```python
from build123d import *

# Parameters (mm, degrees)
SKETCH1_R           = 57.15
SKETCH1_R_2         = 48.26
BOSS_EXTRUDE1_DEPTH = 8.89
SKETCH1_4_R         = 57.15
SKETCH1_4_R_2       = 48.26
BOSS_EXTRUDE2_DEPTH = 177.8
FILLET1_R           = 5


with BuildPart() as part:
    # Sketch1 → Boss-Extrude1 (new body)
    with BuildSketch(Plane(origin=(0, 0, 0), x_dir=(1, 0, 0), z_dir=(0, 1, 0))):
        with Locations(Location((0, 0, 0), (0, 0, 90))):
            Circle(SKETCH1_R)
        Circle(SKETCH1_R_2, mode=Mode.SUBTRACT)
        Circle(SKETCH1_R_2)
    extrude(amount=BOSS_EXTRUDE1_DEPTH)

    # Sketch1_4 → Boss-Extrude2 (add)
    with BuildSketch(Plane(origin=(0, 0, 0), x_dir=(1, 0, 0), z_dir=(0, 1, 0))):
        with Locations(Location((0, 0, 0), (0, 0, 90))):
            Circle(SKETCH1_4_R)
        with Locations(Location((0, 0, 0), (0, 0, 270))):
            Circle(SKETCH1_4_R_2, mode=Mode.SUBTRACT)
    extrude(amount=BOSS_EXTRUDE2_DEPTH)

    # Fillet1
    fillet1_edges = [part.edges().sort_by_distance(p)[0] for p in [
        (0, 0, 57.15),
        (0, 177.8, 57.15),
    ]]
    fillet(fillet1_edges, radius=FILLET1_R)


solid = part.part
```
Check sheet for the modelled part. Datum: model origin and axes. Units: mm. A direction names the side the tool comes from. Round coordinates to 2 decimals unless told otherwise and drop trailing zeros. Order: outer loops, then holes, each group sorted by start corner. A loop starts at its lowest first (then second) coordinate and runs counter-clockwise, first axis right, second up.
1) Scan lines: line 1 (X direction, y = 76, z = 0); line 2 (X direction, y = 62, z = 1); line 3 (Y direction, x = 10, z = 28.5). Record each from-to range of solid material in increasing order.
2) Tool access check on faces 4 (the flat face through (46.1, 177.8, -15.2)), 5 (the cylindrical face through (14.5, 92.16, 46.03)). Record the directions out of +Z, -Z, +X, -X, +Y, -Y that give a thin tool (end or side, any length) a straight path to the whole face; none if there is none.
3) Go/stop test with flat-tipped pins: pin 1 Ø8 at (x, y) = (-18, 137.5) entering from -Z; pin 2 Ø8 at (y, z) = (53.5, 3.5) entering from +X; pin 3 Ø6 at (x, z) = (41.5, 42) entering from +Y. Record where each tip stops, or that it passes through.
4) Section check C-C (y = 45.5). Record the boundary of the cut face in (x, z), and give its area (3 significant figures).
5) Section check A-A (x = 0). Record the boundary of the cut face in (y, z).
6) Section check B-B (z = 0). Record the boundary of the cut face in (x, y).
7) Mould release check, pull along Z, two halves, no side actions. Record for faces 1 (the flat face through (-1, 8.89, 1)), 2 (the flat face through (-1, 0, 1)), 3 (the cylindrical face through (-2.513, 87.725, 57.095)): +Z half, -Z half, draft (parallel to the pull), parting line (faces both ways), or undercut.
Result:
1. line 1: x = -57.15 to -48.26, 48.26 to 57.15
1. line 2: x = -57.14 to -48.25, 48.25 to 57.14
1. line 3: y = 0 to 8.89
2. face 4: +Z, -Z, +X, -X, +Y
2. face 5: +Y
3. pin 1: stops at z = -55.41
3. pin 2: stops at x = 57.15
3. pin 3: stops at y = 175.94
4. outline: circle Ø114.3 at (0, 0); hole circle Ø96.52 at (0, 0)
4. area: 2,940 mm2
5. outline: (0, -52.15) arc R5 ccw to (5, -57.15) - (172.8, -57.15) arc R5 ccw to (177.8, -52.15) - (177.8, -48.26) - (8.89, -48.26) - (8.89, 48.26) - (177.8, 48.26) - (177.8, 52.15) arc R5 ccw to (172.8, 57.15) - (5, 57.15) arc R5 ccw to (0, 52.15) - close
6. outline: (-57.15, 5) arc R5 ccw to (-52.15, 0) - (52.15, 0) arc R5 ccw to (57.15, 5) - (57.15, 172.8) arc R5 ccw to (52.15, 177.8) - (48.26, 177.8) - (48.26, 8.89) - (-48.26, 8.89) - (-48.26, 177.8) - (-52.15, 177.8) arc R5 ccw to (-57.15, 172.8) - close
7. face 1: undercut
7. face 2: draft
7. face 3: parting line
